Autodesk Inventor part; units mm, degrees
ref_plane "YZ Plane" through (0, 0, 0) normal (1, 0, 0) x (0, 1, 0)
ref_plane "XZ Plane" through (0, 0, 0) normal (0, 1, 0) x (-1, 0, 0)
ref_plane "XY Plane" through (0, 0, 0) normal (0, 0, 1) x (1, 0, 0)
sketch "Sketch1" plane through (0, 0, 0) normal (0, 0, 1) x (1, 0, 0)
  circle A0 centre (0, 0) radius 50
  circle A1 centre (0, 0) radius 11
  circle A2 centre (0, 0) radius 57.5
  dimension "d0" = 100
  dimension "d1" = 22
  dimension "d2" = 115
extrude "Extrusion7" add sketch "Sketch1" along normal blind 17.5 and the other way blind 2.5 contours A0
extrude "Extrusion8" add sketch "Sketch1" along normal blind 17.5 and the other way blind 2.5
extrude "Extrusion9" cut sketch "Sketch1" along normal blind 15 contours A2
extrude "Extrusion10" cut sketch "Sketch1" along normal blind 20 and the other way blind 10 contours A1
sketch "Sketch5" plane through (0, 0, -2.5) normal (0, 0, -1) x (-1, 0, 0)
  circle A0 centre (0, 0) radius 40
  line L0 (0, 40) -> (1, 40)
  line L1 (1, 40) -> (1, 43)
  line L2 (0, 44) -> (0, 40)
  line L3 (7, 46) -> (7, 45)
  line L4 (7, 45) -> (3, 45)
  arc A1 (3, 45) -> (1, 43) centre (3, 43) ccw
  arc A2 (2, 46) -> (0, 44) centre (2, 44) ccw
  line L5 (2, 46) -> (7, 46)
  dimension "d35" = 80
  dimension "d37" = 1
  dimension "d38" = 4
  dimension "d39" = 2
  dimension "d40" = 2
  dimension "d41" = 1
  dimension "d42" = 7
extrude "Extrusion11" cut sketch "Sketch5" against normal blind 8
sketch "Sketch6" plane through (0, 0, 0) normal (0, 1, 0) x (-1, 0, 0)
  circle A0 centre (0, 0) radius 4
  dimension "d45" = 8
extrude "Extrusion12" cut sketch "Sketch6" against normal blind 77.25
properties part number "Return_Spool"
Source: CAD feature listing. Evaluate the final solid. Frame: model axes, mm. A direction names the side the tool comes from. Give positions to 0.01 mm unless a question says otherwise; leave off trailing zeros. Write each loop counter-clockwise with the first axis right and the second up, starting at its lowest first coordinate (ties: lowest second). Pieces come first, ordered by that corner, then holes. Notation, with made-up numbers: (-28, -22) -> (-22, -22) arc R27 ccw to (-22, 2) -> close; hole circle Ø5 at (17.5, 21). An arc over 180 degrees is marked (long way). Write item = value, one per line.
Q1. Line query: line 1 (Z direction, x = -5.5, y = 52); line 2 (X direction, y = 0, z = 9.5). Output: solid intervals per line, ascending. Write a range as from..to.
Here are the results:
line_1 = -2.5..0, 15..17.5
line_2 = -50..-11, 11..50
Q2. Cut plane C-C on y = -31. Return loops of the section in (x, z).
Here are the results:
outline = (-48.43, -2.5) -> (-25.28, -2.5) -> (-25.28, 5.5) -> (25.28, 5.5) -> (25.28, -2.5) -> (48.43, -2.5) -> (48.43, 0) -> (39.23, 0) -> (39.23, 15) -> (48.43, 15) -> (48.43, 17.5) -> (-48.43, 17.5) -> (-48.43, 15) -> (-39.23, 15) -> (-39.23, 0) -> (-48.43, 0) -> close
Q3. Cut plane B-B on x = 35.5. Return loops of the section in (y, z), then the cut area to 3 significant figures.
Here are the results:
outline = (-45.23, -2.5) -> (-18.43, -2.5) -> (-18.43, 5.5) -> (18.43, 5.5) -> (18.43, -2.5) -> (45.23, -2.5) -> (45.23, 0) -> (35.21, 0) -> (35.21, 15) -> (45.23, 15) -> (45.23, 17.5) -> (-45.23, 17.5) -> (-45.23, 15) -> (-35.21, 15) -> (-35.21, 0) -> (-45.23, 0) -> close
area = 1,210 mm²
Q4. Reachability of faces 1 (the face through (34, -38, 0)), 2 (the face through (-39, -12, -2.5)), 3 (the face through (-5, 45, 1)), 4 (the face through (0, -47, 4)) from +Z, -Z, +X, -X, +Y, -Y: full face, straight path, thin tool, end or side. Return the list, or none.
Here are the results:
face_1 = none
face_2 = -Z, +X, -X, +Y, -Y
face_3 = -Z
face_4 = -Y
Q5. First-contact query: pin 1 (5 mm diameter, centred on y = 45.5, z = 9.5, fed in from -X); pin 2 (0.8 mm diameter, centred on y = 45.5, z = 1.5, fed in from +X); pin 3 (3 mm diameter, centred on x = 36, z = 10, fed in from +Y); pin 4 (17.5 mm diameter, centred on x = 0, y = 0, fed in from +Z). Flat tips, straight axial feed; report the tip coordinate or a pass-through.
Here are the results:
pin_1 = -25.51
pin_2 = 21.59
pin_3 = 36.19
pin_4 = through
Q6. Mould query, pull axis Y, two halves, no side actions, for faces 5 (the face through (47.69, -15.02, 7.4)), 6 (the face through (-17.3, 47.1, 15)), 7 (the face through (-2, 45, 5.5)). Classes: +Y half, -Y half, draft (parallel to the pull), parting line (faces both ways), or undercut.
Here are the results:
face_5 = parting line
face_6 = draft
face_7 = undercut
Q7. Cut plane A-A on z = 11.5. Return loops of the section in (x, y).
Here are the results:
outline = circle Ø100 at (0, 0); hole circle Ø22 at (0, 0)
